Autodesk Inventor part; units mm, degrees
ref_plane "YZ Plane" through (0, 0, 0) normal (1, 0, 0) x (0, 1, 0)
ref_plane "XZ Plane" through (0, 0, 0) normal (0, 1, 0) x (-1, 0, 0)
ref_plane "XY Plane" through (0, 0, 0) normal (0, 0, 1) x (1, 0, 0)
sketch "Sketch1" plane through (0, 0, 0) normal (0, 1, 0) x (-1, 0, 0)
  line L0 (0, 0) -> (31.75, 0)
  line L1 (31.75, 0) -> (31.75, -76.2)
  line L2 (31.75, -76.2) -> (0, -76.2)
  line L3 (0, -76.2) -> (0, 0)
  line L4 (31.75, -131.1926) -> (0, -131.1926)
  line L5 (0, -131.1926) -> (-15.875, -103.6963)
  line L6 (-15.875, -103.6963) -> (0, -76.2)
  line L7 (0, -76.2) -> (31.75, -76.2)
  line L8 (31.75, -76.2) -> (47.625, -103.6963)
  line L9 (47.625, -103.6963) -> (31.75, -131.1926)
  line L10 (10.3741, -98.1972) -> (21.3741, -98.1972)
  line L11 (21.3741, -98.1972) -> (21.3741, -109.1972)
  line L12 (21.3741, -109.1972) -> (10.3741, -109.1972)
  line L13 (10.3741, -109.1972) -> (10.3741, -98.1972)
  circle A0 centre (21.3741, -98.1972) radius 1.8034
  circle A1 centre (21.3741, -109.1972) radius 1.8034
  circle A2 centre (10.3741, -109.1972) radius 1.8034
  circle A3 centre (10.3741, -98.1972) radius 1.8034
  line L14 (15.875, -131.1926) -> (15.875, -76.2)
  line L15 (47.625, -103.6963) -> (-15.875, -103.6963)
  line L16 (19.685, -85.8288) -> (12.065, -85.8288)
  line L17 (12.065, -85.8288) -> (12.065, -95.9888)
  line L18 (12.065, -95.9888) -> (19.685, -95.9888)
  line L19 (19.685, -95.9888) -> (19.685, -85.8288)
  point P0 (15.875, -103.6963)
  point P1 (15.8741, -98.1972)
  point P2 (31.75, -76.2)
  point P3 (0, -76.2)
  dimension "d0" = 31.75
  dimension "d1" = 76.2
  dimension "d65" = 31.75
  dimension "d66" = 11
  dimension "d67" = 11
  dimension "d68" = 5.4991
  dimension "d69" = 5.4991
  dimension "d70" = 3.6068
  dimension "d71" = 3.6068
  dimension "d72" = 3.6068
  dimension "d73" = 3.6068
  dimension "d94" = 10.16
  dimension "d96" = -1.6909
  dimension "d97" = 7.62
  dimension "d98" = 3.81
extrude "Extrusion1" add sketch "Sketch1" along normal blind 6.35 contours L0 L1 L2 L3 | L2 L14 L16 L17 L18 L10 A3 L13 L15 L6 | L8 L15 L11 A0 L10 L14 L18 L19 L16 L2 | L15 L13 A2 L12 L14 L4 L5 | L9 L4 L14 L12 A1 L11 L15 | L15 L14 L12 A2 L13 | L13 A3 L10 L14 L15 | L15 L14 L10 A0 L11 | L11 A1 L12 L14 L15
sketch "Sketch4" plane through (0, 6.35, 0) normal (0, 1, 0) x (1, 0, 0)
  circle A0 centre (-7.62, 8.89) radius 2.667
  line L0 (-31.75, 0) -> (0, 0)
  line L1 (0, 0) -> (0, 76.2)
  circle A1 centre (-24.13, 8.89) radius 2.667
  line L2 (-31.75, 76.2) -> (-31.75, 0)
  point P0 (0, 127)
  point P1 (-31.75, 127)
  dimension "d11" = 5.334
  dimension "d12" = 8.89
  dimension "d13" = 7.62
  dimension "d14" = 5.334
  dimension "d15" = 8.89
  dimension "d16" = 7.62
extrude "Extrusion4" cut sketch "Sketch4" against normal blind 36.5125
sketch "Sketch8" plane through (0, 6.35, 0) normal (0, 1, 0) x (1, 0, 0)
  circle A0 centre (-10.3741, 98.1972) radius 1.8034
  circle A1 centre (-10.3741, 109.1972) radius 1.8034
  circle A2 centre (-21.3741, 109.1972) radius 1.8034
  circle A3 centre (-21.3741, 98.1972) radius 1.8034
  line L0 (0, 0) -> (0, 76.2)
  line L1 (0, 76.2) -> (15.875, 103.6963)
  line L2 (15.875, 103.6963) -> (0, 131.1926)
  line L3 (0, 131.1926) -> (-31.75, 131.1926)
  line L4 (-31.75, 131.1926) -> (-47.625, 103.6963)
  line L5 (-47.625, 103.6963) -> (-31.75, 76.2)
  line L6 (-31.75, 76.2) -> (-31.75, 0)
  line L7 (-30.0159, 27.1341) -> (-1.7341, 27.1341)
  line L8 (-1.7341, 27.1341) -> (-1.7341, 76.6646)
  line L9 (-1.7341, 76.6646) -> (13.8726, 103.6963)
  line L10 (13.8726, 103.6963) -> (-1.0012, 129.4585)
  line L11 (-1.0012, 129.4585) -> (-30.7488, 129.4585)
  line L12 (-30.7488, 129.4585) -> (-45.6226, 103.6963)
  line L13 (-45.6226, 103.6963) -> (-30.0159, 76.6646)
  line L14 (-30.0159, 76.6646) -> (-30.0159, 27.1341)
  line L15 (-31.75, 0) -> (0, 0)
extrude "Extrusion7" cut sketch "Sketch8" against normal blind 1.5875 contours L14 L13 L12 L11 L10 L9 L8 L7
sketch "Sketch9" plane through (-1.7341, 6.35, -27.1341) normal (0, 0, -1) x (-1, 0, 0)
  line L0 (0, 0) -> (28.2818, 0)
  line L1 (0, 0) -> (0, -1.5875)
  line L2 (0, -1.5875) -> (28.2818, -1.5875)
  line L3 (28.2818, 0) -> (28.2818, -1.5875)
  line L4 (30.0159, 0) -> (-1.7341, 0)
  line L5 (14.1409, 0) -> (14.1409, -1.5875)
  line L6 (21.2148, 0) -> (24.3898, 0)
  line L7 (-1.7341, -3.175) -> (30.0159, -3.175)
  line L8 (21.2148, 0) -> (18.0398, 0)
  line L9 (18.0398, 0) -> (18.0398, -1.5875)
  line L10 (24.3898, 0) -> (24.3898, -1.5875)
  line L11 (28.2818, 0) -> (0, 0)
  line L12 (-1.7341, 0) -> (30.0159, 0)
  line L13 (7.067, 0) -> (3.892, 0)
  line L14 (7.067, 0) -> (10.242, 0)
  line L15 (10.242, 0) -> (10.242, -1.5875)
  line L16 (3.892, 0) -> (3.892, -1.5875)
  point P0 (-1.7341, -6.35)
  point P1 (14.1409, -0.7937)
  point P2 (3.892, 0)
  point P3 (3.892, -1.5875)
  point P4 (10.242, 0)
  dimension "d79" = 7.0739
  dimension "d80" = 3.175
  dimension "d82" = 3.175
extrude "Extrusion8" add sketch "Sketch9" along normal blind 49.2125 contours L0 L15 L2 L16 | L0 L10 L2 L9
fillet "Fillet2" radius 3.175 2 edges at (-8.8011, 6.35, -76.3466) (-22.9489, 6.35, -76.3466)
fillet "Fillet4" radius 3.175 4 edges at (-45.6226, 5.5562, -103.6963) (13.8726, 5.5562, -103.6963) (-30.7488, 5.5562, -129.4585) (-1.0012, 5.5562, -129.4585)
ref_plane "Work Plane1" through (0, 3.175, 0) normal (0, 1, 0) x (1, 0, 0)
sketch "Sketch11" plane through (0, 3.175, 0) normal (0, 1, 0) x (1, 0, 0)
  line L0 (-0.0667, 22.8993) -> (-31.8167, 22.8612)
  line L1 (0, 25.4) -> (0, 0)
  line L2 (-31.75, 25.4) -> (0, 25.4)
  line L3 (-31.75, 0) -> (-31.75, 25.4)
  line L4 (0, 25.4) -> (-31.75, 25.4)
  line L5 (-31.75, 25.4) -> (-31.75, 22.8613)
  line L6 (-31.75, 22.8613) -> (0, 22.8613)
  line L7 (0, 22.8613) -> (0, 25.4)
extrude "Extrusion9" add sketch "Sketch11" along normal blind 3.175
sketch "Sketch13" plane through (0, 6.35, 0) normal (0, 1, 0) x (1, 0, 0)
  line L0 (-1.1058, 21.2778) -> (-31.081, 21.2778)
  line L1 (-31.081, 21.2778) -> (-31.081, 31.4378)
  line L2 (-31.081, 31.4378) -> (-1.1058, 31.4378)
  line L3 (-1.1058, 31.4378) -> (-1.1058, 21.2778)
  point P0 (0, 0)
  dimension "d99" = 10.16
extrude "Extrusion11" add sketch "Sketch13" against normal blind 3.175
sketch "Sketch14" plane through (-31.75, 0, -76.2) normal (-1, 0, 0) x (0, 0, 1)
  line L0 (44.7622, 6.35) -> (53.3387, 6.35)
  line L1 (0, 6.35) -> (76.2, 6.35)
  line L2 (44.7622, 4.7625) -> (-0.1466, 4.7625)
  line L3 (44.7622, 6.35) -> (2.603, 6.35)
  line L4 (53.3387, 6.35) -> (53.3387, 4.7625)
  line L5 (53.3387, 4.7625) -> (34.8482, 4.7625)
  line L6 (53.3387, 6.35) -> (53.3387, 11.938)
  line L7 (53.3387, 11.938) -> (34.8482, 4.7625)
  point P0 (76.2, 0)
  dimension "d107" = 5.588
extrude "Extrusion12" add sketch "Sketch14" against normal blind 31.75
fillet "Fillet9" radius 3.175 7 edges at (-0.867, 6.35, -37.261) (-8.8011, 6.35, -37.261) (-22.9489, 6.35, -37.261) (-30.883, 6.35, -37.261) (-15.875, 4.7625, -41.3518) (-28.0699, 4.7625, -41.3518) (-3.6801, 4.7625, -41.3518)
properties part number "Arm"
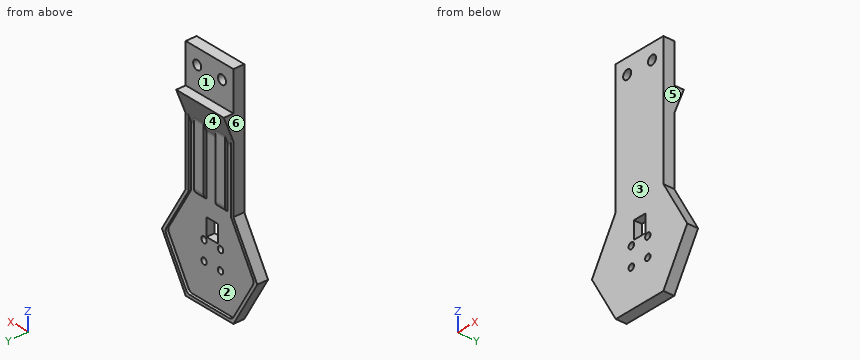
Can you work these out from the model? Positions are in its coordinate system, mm. Face numbers are marked on the shaded views. A direction names the side the tool comes from. Coordinates: 2 decimals unless noted, no trailing zeros. Order: outer loops, then holes, each group sorted by start corner. A loop starts at its lowest first (then second) coordinate and runs counter-clockwise, first axis right, second up. Notation, with made-up numbers: (53, 3) - (82, 3) arc R26 cw to (82, 28) - close; hole circle Ø5 at (44.5, 27.5). An arc over 180 degrees is marked (long way). Answer as a JSON object with one key per item and string values. Group by question number.
Q1. On a 3-axis mill with a long thin cutter (end or side, diameter ignored), from which of +Z, -Z, +X, -X, +Y, -Y can I reach the whole of each face in a straight line? I mean the marked faces 3, 4, 5 and 6. Say none if no direction works.
Q2. Imagine slicing it at D-D (y = 8.25). Please give me the cut outline in (x, z), and give its area (3 significant figures).
Q3. We'd pull the mould along Z, two halves only. Please class the marked faces 1 and 2: +Z half, -Z half, draft (parallel to the pull), parting line (faces both ways), or undercut.
Q4. I need wall thicknesses on line 1 (X direction, y = 5, z = -60.5); line 2 (X direction, y = 3.5, z = -108); line 3 (Z direction, x = -18, y = 1). Which ranges of each line are inside material? Lowest first, please. Write a range as from..to.
Q5. Imagine slicing it at B-B (x = 11.5). Please give me the cut outline in (y, z), and give its area (3 significant figures).
Q6. Imagine slicing it at A-A (z = -8.89). Please give me the cut outline in (x, y).
Q7. Will these pins go through, and if not, where does the flat tip stop? P1, Ø6, axis at y = 5, z = -51.5, coming from the -X side; P2, Ø5, axis at x = -39, y = 7.5, coming from the +Z side; P3, Ø1.9, axis at x = -8.5, z = -56, coming from the +Y side.
Q8. Imagine slicing it at C-C (y = 1.75). Give the number of separate pieces and of enclosed holes in the cut face, and give its area (3 significant figures).
Determined:
{
 "1": {"face 3": "+Z, -Z, +X, -X, -Y", "face 4": "+Y", "face 5": "+Z, +X, +Y, -Y", "face 6": "+Z, -X, +Y, -Y"},
 "2": {"outline": "(-31.75, -32.36) - (0, -32.36) - (0, -22.86) - (-31.75, -22.86) - close", "area": "302 mm2"},
 "3": {"face 1": "draft", "face 2": "undercut"},
 "4": {"line 1": "x = -31.75..-30.02, -26.12..-19.77, -11.98..-5.63, -1.73..0", "line 2": "x = -45.14..-22.72, -20.03..-11.72, -9.03..13.39", "line 3": "z = -131.19..-95.99, -85.83..0"},
 "5": {"outline": "(0, -111.27) - (6.35, -111.27) - (6.35, -107.81) - (4.76, -107.81) - (4.76, -99.59) - (6.35, -99.59) - (6.35, -96.12) - (0, -96.12) - close", "area": "83.2 mm2"},
 "6": {"outline": "(-31.75, 0) - (-26.8, 0) - (-26.8, 6.35) - (-31.75, 6.35) - close; (-21.46, 0) - (-10.29, 0) - (-10.29, 6.35) - (-21.46, 6.35) - close; (-4.95, 0) - (0, 0) - (0, 6.35) - (-4.95, 6.35) - close"},
 "7": {"P1": "stops at x = -31.75", "P2": "stops at z = -84.91", "P3": "stops at y = 6.35"},
 "8": {"separate pieces": "1", "enclosed holes": "7", "area": "4,880 mm2"}
}
